```python
from build123d import *

# Parameters (mm, degrees)
SKETCH_1_W      = 80
SKETCH_1_H      = 27.309222572
SKETCH_1_R      = 1.25
SKETCH_1_W_2    = 22.7
SKETCH_1_H_2    = 12.5
EXTRUDE_2_DEPTH = 4
SKETCH_1_4_R    = 0.5
EXTRUDE_3_DEPTH = 2


with BuildPart() as part:
    # Sketch 1 → Extrude 2 (new body)
    with BuildSketch(Plane(origin=(0, 0, 0), x_dir=(1, 0, 0), z_dir=(0, 1, 0))):
        Rectangle(SKETCH_1_W, SKETCH_1_H)
        with BuildLine():
            ThreePointArc((-34.15, -3.48245603), (-38, 0), (-34.15, 3.48245603))
            Line((-34.15, 3.48245603), (-19.3, 1.989974874))
            ThreePointArc((-19.3, 1.989974874), (-18.016760303, 1.341640786), (-17.5, 0))
            ThreePointArc((-17.5, 0), (-18.016760303, -1.341640786), (-19.3, -1.989974874))
            Line((-19.3, -1.989974874), (-34.15, -3.48245603))
        make_face(mode=Mode.SUBTRACT)
        with Locations(Location((7, 0, 0), (0, 0, 270))):
            Circle(SKETCH_1_R, mode=Mode.SUBTRACT)
        with Locations((20.75, 0)):
            Rectangle(SKETCH_1_W_2, SKETCH_1_H_2, mode=Mode.SUBTRACT)
        with Locations(Location((34.5, 0, 0), (0, 0, 270))):
            Circle(SKETCH_1_R, mode=Mode.SUBTRACT)
    extrude(amount=EXTRUDE_2_DEPTH)

    # Sketch 1_4 → Extrude 3 (add)
    with BuildSketch(Plane(origin=(0, 0, 0), x_dir=(1, 0, 0), z_dir=(0, 1, 0))):
        with BuildLine():
            Line((-19.3, 1.989974874), (-34.15, 3.48245603))
            ThreePointArc((-34.15, 3.48245603), (-38, 0), (-34.15, -3.48245603))
            Line((-34.15, -3.48245603), (-19.3, -1.989974874))
            ThreePointArc((-19.3, -1.989974874), (-17.5, 0), (-19.3, 1.989974874))
        make_face()
        with Locations(Location((-21.5, 0, 0), (0, 0, 270))):
            Circle(SKETCH_1_4_R, mode=Mode.SUBTRACT)
    extrude(amount=EXTRUDE_3_DEPTH)


solid = part.part
```
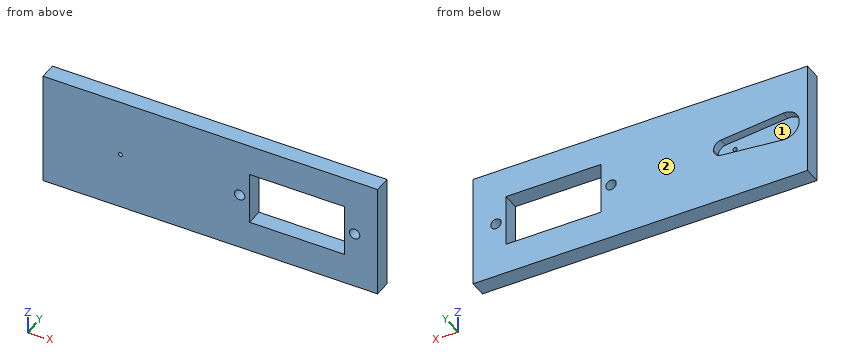
Source: CAD feature listing. Evaluate the final solid. Frame: model axes, mm. Face numbers are marked on the shaded views. Give positions to 0.01 mm unless a question says otherwise; leave off trailing zeros. Order: outer loops, then holes, each group sorted by start corner. A loop starts at its lowest first (then second) coordinate and runs counter-clockwise, first axis right, second up.
(1) Material intervals for line 1 along X through (y, z) = (0.6, 0); line 2 along X through (y, z) = (2.45, 0); line 3 along X through (y, z) = (3.7, 5.25), sorted ascending.
(2) Section query B-B (y = 2.85). Return the cut outline in (x, z).
(3) Contact query for flat-ended pins moving along their axis: P1, Ø12, axis at x = 16.5, z = 5.5, coming from the -Y side; P2, Ø6.5, axis at x = -34.5, z = 0, coming from the +Y side. Output: stop coordinate, or through.
(4) Section query C-C (z = -4.5). Return the cut outline in (x, y), plus the area to 3 significant figures.
(5) Section query D-D (x = -26). Return the cut outline in (y, z), plus the area to 3 significant figures.
(6) Pull-direction query (Z, two-part tool) for the marked faces 1 and 2; classes: +Z half, -Z half, draft (parallel to the pull), parting line (faces both ways), or undercut.
(7) Section query A-A (x = 7). Return the cut outline in (y, z), plus the area to 3 significant figures.
Outcome:
1. line 1: x = -40 to -22, -21 to 5.75, 8.25 to 9.4, 32.1 to 33.25, 35.75 to 40
1. line 2: x = -40 to -38, -17.5 to 5.75, 8.25 to 9.4, 32.1 to 33.25, 35.75 to 40
1. line 3: x = -40 to 9.4, 32.1 to 40
2. outline: (-40, -13.65) - (40, -13.65) - (40, 13.65) - (-40, 13.65) - close; hole (-34.15, -3.48) - (-19.3, -1.99) arc R2 ccw to (-19.3, 1.99) - (-34.15, 3.48) arc R3.5 ccw (long way) to start; hole circle Ø2.5 at (7, 0); hole (9.4, -6.25) - (32.1, -6.25) - (32.1, 6.25) - (9.4, 6.25) - close; hole circle Ø2.5 at (34.5, 0)
3. P1: stops at y = 0
3. P2: stops at y = 2
4. outline: (-40, 0) - (9.4, 0) - (9.4, 4) - (-40, 4) - close; (32.1, 0) - (40, 0) - (40, 4) - (32.1, 4) - close
4. area: 229 mm2
5. outline: (0, -13.65) - (4, -13.65) - (4, -2.66) - (2, -2.66) - (2, 2.66) - (4, 2.66) - (4, 13.65) - (0, 13.65) - close
5. area: 98.6 mm2
6. face 1: undercut
6. face 2: draft
7. outline: (0, -13.65) - (4, -13.65) - (4, -1.25) - (0, -1.25) - close; (0, 1.25) - (4, 1.25) - (4, 13.65) - (0, 13.65) - close
7. area: 99.2 mm2
